Answer from the drawing. Dimensions are ordinates in mm from the lowest x, y and z of the part. Give positions to 0.01 mm unless a question says otherwise; leave off trailing zeros. Write each loop counter-clockwise with the first axis right and the second up, starting at its lowest first coordinate (ties: lowest second). Pieces come first, ordered by that corner, then holes.
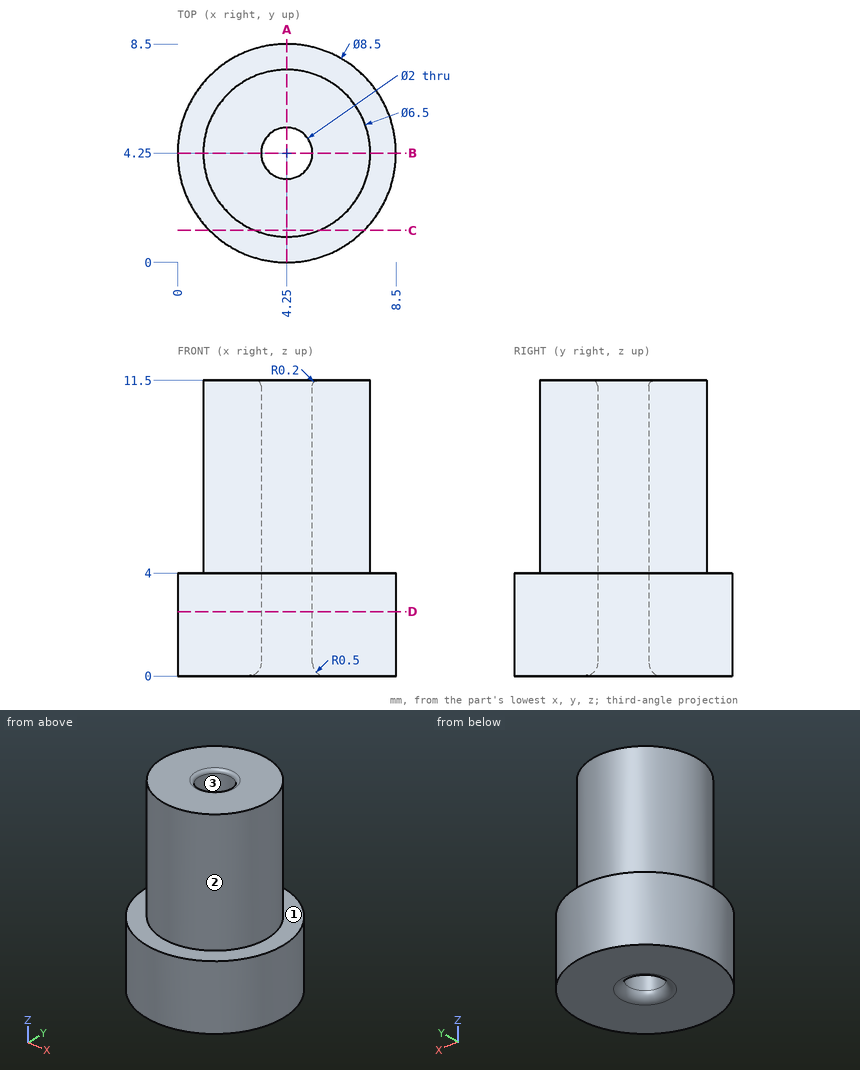
Item 1: Find the intervals of material crossed by line 1 along Y through (x, z) = (4.25, 4.5); line 2 along Z through (x, y) = (7.75, 3.75); line 3 along X through (y, z) = (3.75, 4.25), in increasing order.
Result set:
line 1: y = 1 to 3.25, 5.25 to 7.5
line 2: z = 0 to 4
line 3: x = 1.04 to 3.38, 5.12 to 7.46
Item 2: Each of these flat-tipped pins is pushed along its axis until it touches: pin 1 Ø5 at (x, z) = (7, 8) entering from +Y; pin 2 Ø5 at (y, z) = (1, 8) entering from +X; pin 3 Ø1.5 at (x, z) = (6.5, 3.5) entering from -Y. Where does it stop, or does it pass through?
Result set:
pin 1: stops at y = 7.49
pin 2: stops at x = 7.41
pin 3: stops at y = 0.27
Item 3: Section C-C (y = 1.25) is taken. Write down the section's boundary in (x, z).
Result set:
outline: (1.24, 0) - (7.26, 0) - (7.26, 4) - (5.5, 4) - (5.5, 11.5) - (3, 11.5) - (3, 4) - (1.24, 4) - close
Item 4: Section A-A (x = 4.25) is taken. Write down the section's boundary in (y, z), and give its area (3 significant figures).
Result set:
outline: (0, 0) - (2.75, 0) arc R0.5 ccw to (3.25, 0.5) - (3.25, 11.3) arc R0.2 ccw to (3.05, 11.5) - (1, 11.5) - (1, 4) - (0, 4) - close; (5.25, 0.5) arc R0.5 ccw to (5.75, 0) - (8.5, 0) - (8.5, 4) - (7.5, 4) - (7.5, 11.5) - (5.45, 11.5) arc R0.2 ccw to (5.25, 11.3) - close
area: 59.6 mm2
Item 5: Determine the mould class of the marked faces 1, 2 and 3 for opening direction Y: pulls with the +Y half, pulls with the -Y half, needs draft (parallel to the pull), parting line crosses it, or undercut.
Result set:
face 1: needs draft
face 2: parting line crosses it
face 3: undercut
Item 6: Section D-D (z = 2.5) is taken. Write down the section's boundary in (x, y).
Result set:
outline: circle Ø8.5 at (4.25, 4.25); hole circle Ø2 at (4.25, 4.25)
